The listing builds one solid part. Answer for the finished solid, in the listing's coordinates (mm). A direction names the side the tool comes from. Coordinates: 2 decimals unless noted, no trailing zeros. Order: outer loops, then holes, each group sorted by start corner. A loop starts at its lowest first (then second) coordinate and runs counter-clockwise, first axis right, second up. Notation, with made-up numbers: (-8.5, 80.5) -> (21.5, 80.5) arc R10 cw to (21.5, 96.5) -> close; hole circle Ø9 at (43.5, -37). An arc over 180 degrees is marked (long way). Write item = value, one per line.
from build123d import *

# Parameters (mm, degrees)
CUT_EXTRUDE1_DEPTH      = 195.978637362
CUT_EXTRUDE1_DEPTH_BACK = 195.978637362
SKETCH4_R               = 2.5
CUT_EXTRUDE2_DEPTH      = 151.611328634
CUT_EXTRUDE2_DEPTH_BACK = 151.611328634
SKETCH3_R               = 2.5


with BuildPart() as part:
    # Sketch2 → Revolve1 (revolve)
    with BuildSketch(Plane.XY, mode=Mode.PRIVATE) as revolve1_sk:
        Polygon((0, 6), (-5, 6), (-5, 7.5), (-29, 7.5), (-29, 5), (0, 5), align=None)
    revolve(revolve1_sk.sketch.rotate(Axis((0, 0, 0), (-1, 0, 0)), 90), axis=Axis((0, 0, 0), (-1, 0, 0)))

    # Sketch4 → Cut-Extrude1 (cut, two sides: drawn at the far end of the back side and taken through both)
    with BuildSketch(Plane(origin=(-120.750059673, 87.243462265, 112.748777435), x_dir=(0.8561890359823346, 0.3016571585603837, 0.41945594924010343), z_dir=(0, 0.8118564738851006, -0.5838570593996881)).offset(-CUT_EXTRUDE1_DEPTH_BACK)):
        with Locations(Location((10.081768965, 172.488088347, 0), (0, 0, 301.108656356))):
            Circle(SKETCH4_R)
    extrude(amount=CUT_EXTRUDE1_DEPTH + CUT_EXTRUDE1_DEPTH_BACK, mode=Mode.SUBTRACT)

    # Sketch3 → Cut-Extrude2 (cut, two sides: drawn at the far end of the back side and taken through both)
    with BuildSketch(Plane(origin=(-120.750059673, -67.453558659, 42.35137307), x_dir=(-0.5093963915480642, 0.6986284720029967, -0.5024276807507421), z_dir=(0, -0.5838570593996879, -0.8118564738851008)).offset(-CUT_EXTRUDE2_DEPTH_BACK)):
        with Locations(Location((14.02538357, 132.353637021, 0), (0, 0, 30.623632048))):
            Circle(SKETCH3_R)
    extrude(amount=CUT_EXTRUDE2_DEPTH + CUT_EXTRUDE2_DEPTH_BACK, mode=Mode.SUBTRACT)


solid = part.part
Q1. Each of these flat-tipped pins is pushed along its axis until it touches: pin 1 Ø6 at (x, y) = (-7.5, 3.5) entering from +Z; pin 2 Ø1 at (x, y) = (-14, -5) entering from -Z; pin 3 Ø4 at (y, z) = (-2, -2.5) entering from +X; pin 4 Ø3 at (x, z) = (-16.5, -4) entering from -Y. Where does it stop, or does it pass through?
The answers:
pin_1 = 7.48
pin_2 = -3.37
pin_3 = 0
pin_4 = -7.07
Q2. The mould has two halves that part along Y. Classify faces 1 (the face through (-17.168, -6.324, -4.032)), 2 (the face through (-29, 5, -2)), 3 (the face through (-14.96, 5.34, 3.47)): released by +Y, released by -Y, zero draft, split by the parting line, or undercut.
The answers:
face_1 = split by the parting line
face_2 = zero draft
face_3 = undercut
Q3. A tool of negligible diameter and unlimited length cuts with its end or side. For faces 4 (the face through (-5, -6, 2)), 5 (the face through (0, -4, -4)), from which of +Z, -Z, +X, -X, +Y, -Y can it reach the whole face along a straight path? Write none if from no direction.
The answers:
face_4 = +X
face_5 = +Z, -Z, +X, +Y, -Y
Q4. Section C-C, the plane x = -3 is taken. Give the vertices of the cut face in (y, z), plus the area to 3 significant figures.
The answers:
outline = circle Ø12 at (0, 0); hole circle Ø10 at (0, 0)
area = 34.6 mm2
Q5. Section A-A, the plane z = 0 is taken. Give the vertices of the cut face in (x, y).
The answers:
outline = (-29, -7.5) -> (-5, -7.5) -> (-5, -6) -> (0, -6) -> (0, -5) -> (-29, -5) -> close; (-29, 5) -> (0, 5) -> (0, 6) -> (-5, 6) -> (-5, 7.5) -> (-29, 7.5) -> close
Q6. Section D-D, the plane z = 3 is taken. Give the number of separate pieces and of enclosed holes in the cut face, plus the area to 3 significant figures.
The answers:
separate_pieces = 3
enclosed_holes = 0
area = 133 mm2
Q7. Find the intervals of material crossed by line 1 along Y through (x, z) = (-21, 0); line 2 along Z through (x, y) = (-20.25, -0.25); line 3 along X through (y, z) = (-5.5, 4), in increasing order.
The answers:
line_1 = -7.5 to -5, 5 to 7.5
line_2 = -7.5 to -4.99, 4.99 to 7.5
line_3 = -29 to -25.5, -20.5 to -5
